Design review of the part shown in the three views and the two pictorial views. Dimensions are in mm from the part's minimum x, y and z. A direction names the side the tool comes from. Coordinates: 2 decimals unless noted, no trailing zeros. Order: outer loops, then holes, each group sorted by start corner. A loop starts at its lowest first (then second) coordinate and runs counter-clockwise, first axis right, second up. Notation, with made-up numbers: (15.5, 18.5) - (43.5, 18.5) arc R15 cw to (43.5, 31.5) - close; hole circle Ø11 at (81, 72). An arc over 180 degrees is marked (long way). One line per item, written item: value. Start each with the question number.
(1) Consider section D-D on y = 11.25. Write out the cut boundary in (x, z).
(2) Mouldability with a two-part tool opening along Z and no side actions: class the marked faces 1, 2 and 3 as released by +Z, released by -Z, zero draft, split by the parting line, or undercut.
(3) Consider section B-B on x = 5.5. Write out the cut boundary in (y, z), then the cut area to 4 significant figures.
(4) Consider section C-C on z = 36. Write out the cut boundary in (x, y), then the cut area to 3 significant figures.
(5) Consider section A-A on y = 6. Write out the cut boundary in (x, z).
(6) Clearance check with flat-ended pins moving along their axes: pin 1 (3 mm diameter, centred on x = 14.5, y = 15, fed in from +Z); pin 2 (5 mm diameter, centred on x = 6, y = 17, fed in from -Z); pin 3 (2.5 mm diameter, centred on x = 43.5, z = 4.7, fed in from -Y); pin 4 (2.5 mm diameter, centred on x = 29.5, z = 40, fed in from +Y). State where each tip first meets the part, or that it passes through.
(7) To check wall thickness, follow line 1 along X through (y, z) = (1, 4.7); line 2 along Z through (x, y) = (43.5, 0.8); line 3 along X through (y, z) = (3, 27.5). State the ranges of each line that lie inside material, in increasing order.
(8) For the marked faces 4, 5, 6, 7 and 8, list the 3-axis set-ups (+Z, -Z, +X, -X, +Y, -Y) from which the entire face can be reached by the end or side of a thin tool; tool diameter is ignored.
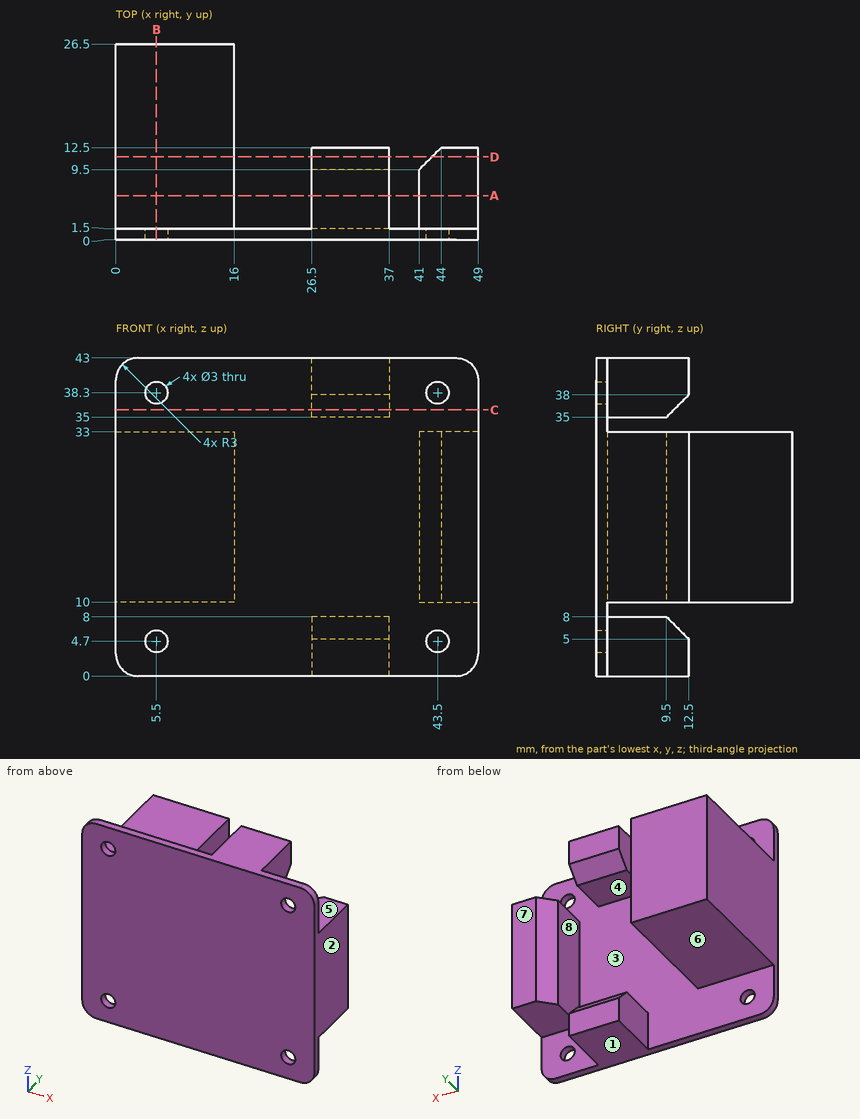
Geometry check:
1. outline: (0, 10) - (16, 10) - (16, 33) - (0, 33) - close; (26.5, 0) - (37, 0) - (37, 6.25) - (26.5, 6.25) - close; (26.5, 36.75) - (37, 36.75) - (37, 43) - (26.5, 43) - close; (42.75, 10) - (49, 10) - (49, 33) - (42.75, 33) - close
2. face 1: released by -Z
2. face 2: zero draft
2. face 3: undercut
3. outline: (0, 0) - (1.5, 0) - (1.5, 3.2) - (0, 3.2) - close; (0, 6.2) - (1.5, 6.2) - (1.5, 10) - (26.5, 10) - (26.5, 33) - (1.5, 33) - (1.5, 36.8) - (0, 36.8) - close; (0, 39.8) - (1.5, 39.8) - (1.5, 43) - (0, 43) - close
3. area: 630.5 mm^2
4. outline: (0, 0) - (49, 0) - (49, 1.5) - (37, 1.5) - (37, 10.5) - (26.5, 10.5) - (26.5, 1.5) - (0, 1.5) - close
4. area: 168 mm^2
5. outline: (0, 10) - (16, 10) - (16, 33) - (0, 33) - close; (26.5, 0) - (37, 0) - (37, 8) - (26.5, 8) - close; (26.5, 35) - (37, 35) - (37, 43) - (26.5, 43) - close; (41, 10) - (49, 10) - (49, 33) - (41, 33) - close
6. pin 1: stops at z = 33
6. pin 2: stops at z = 10
6. pin 3: passes through
6. pin 4: stops at y = 12.5
7. line 1: x = 0 to 4, 7 to 42, 45 to 49
7. line 2: z = 0 to 3.2, 6.2 to 36.8, 39.8 to 43
7. line 3: x = 0 to 16, 41 to 49
8. face 4: +X, -X, +Y
8. face 5: +Z, +X, -X, +Y
8. face 6: -Z, +X, -X, +Y
8. face 7: +Z, -Z, +X, +Y
8. face 8: +Z, -Z, +Y
